Autodesk Inventor part; units mm, degrees
ref_plane "WorkPlane1" through (0, 0, 0) normal (0, 0, 1) x (1, 0, 0)
ref_plane "MSC_PF1" through (0, 0, 0) normal (1, 0, 0) x (0, 1, 0)
ref_plane "MSC_PT1" through (0, 0, 0) normal (0, 0, -1) x (-1, 0, 0)
ref_plane "WorkPlane1" through (0, 0, 0) normal (0, 0, 1) x (1, 0, 0)
sketch "Sketch1" plane through (0, 0, 0) normal (0, 0, 1) x (1, 0, 0)
  point P0 (0, 0)
sketch "Sketch2" plane through (0, 0, 0) normal (0, 0, 1) x (1, 0, 0)
  line L0 (-5, 2.8868) -> (-5, -2.8868)
  line L1 (0, 5.7734) -> (-5, 2.8868)
  line L2 (5, 2.8868) -> (0, 5.7734)
  line L3 (5, -2.8868) -> (5, 2.8868)
  line L4 (0, -5.7734) -> (5, -2.8868)
  line L5 (-5, -2.8868) -> (0, -5.7734)
  circle A0 centre (0, 0) radius 5 construction
  dimension "d1" = 10
  dimension "d29" = 0
  dimension "d30" = 0
extrude "Extrusion1" add sketch "Sketch2" along normal blind 4
sketch "Sketch3" plane through (0, 0, 0) normal (1, 0, 0) x (0, 1, 0)
  line L0 (5, 4) -> (5.8734, 4)
  line L1 (5.8734, 3.4957) -> (5, 4)
  line L2 (5.8734, 4) -> (5.8734, 3.4957)
  line L3 (0, -0.8) -> (0, 4.8)
  line L4 (5.7734, 0) -> (5.7734, 4)
  dimension "d25" = 0.1
  dimension "d26" = 0
  dimension "d27" = 60
  dimension "d28" = 5
revolve "Revolution1" cut sketch "Sketch3" angle 360 about axis through (0, 0, -10) along (0, 0, 1)
sketch "Sketch4" plane through (0, 0, 0) normal (1, 0, 0) x (0, 1, 0)
  line L0 (0, -30) -> (0, 0)
  line L1 (-3, -30) -> (0, -30)
  line L2 (-3, 0) -> (-3, -30)
  line L3 (0, 0) -> (-3, 0)
  line L4 (0, -30) -> (0, 0)
  line L5 (-3.6, 0) -> (0.6, 0)
  line L6 (0, -36) -> (0, 6)
  dimension "d18" = 3
  dimension "d20" = 30
  dimension "d33" = 0
  dimension "d34" = 0
revolve "Revolution2" add sketch "Sketch4" angle 360 about axis through (0, 0, -30) along (0, 0, -1)
chamfer "Chamfer1" distance 0.5 angle 45 1 edges at (0, 3, -30)
fillet "Fillet1" radius 0.25 1 edges at (0, 3, 0)
thread "Thread1"
ref_plane "MSC_PF1" through (0, 0, 0) normal (1, 0, 0) x (0, 1, 0)
ref_plane "MSC_PT1" through (0, 0, 0) normal (0, 0, -1) x (-1, 0, 0)
equation "\"d22\" = 0.5 * PTC"
equation "\"d23\" = 0.5 * PTC"
equation "\"d24\" = r"
equation "\"d1\" = ParS"
equation "\"d6\" = ParK"
equation "\"d28\" = 0.5 * ParS"
equation "\"d18\" = 0.5 * NND"
equation "\"d20\" = NLG"
equation "\"NND\" = 6"
equation "\"NLG\" = 30"
equation "\"PTC\" = 1"
equation "\"ParK\" = 4"
equation "\"ParS\" = 10"
equation "\"msp_es\" = 0.577367 * ParS"
equation "\"r\" = 0.25"
equation "\"THREADDIA\" = NND"
properties part number "ISO 4016 - M6 x 30" material "Steel"
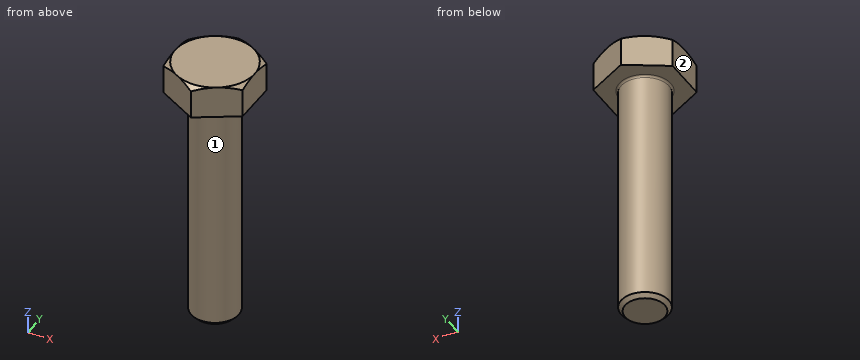
Check sheet for the modelled part. Datum: model origin and axes. Units: mm. Face numbers are marked on the shaded views. A direction names the side the tool comes from. Coordinates: 2 decimals unless noted, no trailing zeros. Order: outer loops, then holes, each group sorted by start corner. A loop starts at its lowest first (then second) coordinate and runs counter-clockwise, first axis right, second up. Notation, with made-up numbers: (18.5, 60) -> (57.5, 60) arc R22 cw to (57.5, 83) -> close; hole circle Ø4 at (-12, 5). An arc over 180 degrees is marked (long way). Write item = value, one per line. Start each with the question number.
1) Access from +Z, -Z, +X, -X, +Y, -Y to the whole of each face (thin tool, end or side, straight path). Record for the marked faces 1 and 2.
2) Go/stop test with flat-tipped pins: P1, Ø1.5, axis at x = 0.5, z = -17, coming from the +Y side; P2, Ø1.5, axis at y = 2, z = -8.5, coming from the +X side. Record where each tip stops, or that it passes through.
3) Cross-section at A-A (z = -3). Enter the section's corners in (x, y), then the cut area to 3 significant figures.
4) Material ranges on L1, parallel to Y at x = 0, z = -22.5; L2, parallel to Z at x = -0.75, y = 3.25; L3, parallel to Y at x = 1.25, z = -2.5, recorded low to high.
Ans:
q1.face_1 = -Z
q1.face_2 = +Z, -Z, -X, +Y, -Y
q2.P1 = 3
q2.P2 = 2.73
q3.outline = circle Ø6 at (0, 0)
q3.area = 28.3 mm²
q4.L1 = -3 to 3
q4.L2 = 0 to 4
q4.L3 = -2.73 to 2.73
